Could you check a few things on this drawing? It's one solid part, dimensions in mm from its lowest x, y, z. A direction names the side the tool comes from. Round coordinates to 2 decimals unless told otherwise and drop trailing zeros. Order: outer loops, then holes, each group sorted by start corner. A loop starts at its lowest first (then second) coordinate and runs counter-clockwise, first axis right, second up. Notation, with made-up numbers: (-29, -17) -> (-6, -17) arc R10 ccw to (-6, -3) -> close; hole circle Ø5 at (59, 32). An arc over 180 degrees is marked (long way). Use a Markdown table: item, result. Add a question column.
(1) If I drill on probe 1 along Y at (x, z) = (6, 1); probe 2 along Y at (x, z) = (20, 7.75) (1 decimal); probe 3 along Y at (x, z) = (21, 3.75), over which ranges is the centre line in solid material (lowest first)?
(2) I want a section at C-C, the plane x = 14.5. Please give me the cut outline in (y, z) (1 decimal), then the cut area to 3 significant figures.
(3) I'm going to push flat-ended pins straight in: P1, Ø3, axis at x = 15, y = 24, coming from the +Z side; P2, Ø1.4, axis at x = 8.5, z = 1.5, coming from the -Y side; P3, Ø4, axis at y = 16.5, z = 3, coming from the -X side; P4, Ø4, axis at x = 11.5, y = 23, coming from the +Z side (1 decimal). Where does each tip first touch, or does it pass through?
(4) Thinking about a two-plate mould opening in Y: for the marked faces 5, 6, 7 and 8, which applies, pulls with the +Y half, pulls with the -Y half, needs draft (parallel to the pull), parting line crosses it, or undercut?
(5) On a 3-axis mill with a long thin cutter (end or side, diameter ignored), from which of +Z, -Z, +X, -X, +Y, -Y can I reach the whole of each face in a straight line? I mean the marked faces 1, 2, 3 and 4. Say none if no direction works.
(6) I want a section at A-A, the plane x = 29.5. Please give me the cut outline in (y, z).
(7) I want a section at B-B, the plane z = 11.5. Please give me the cut outline in (x, y) (1 decimal), then the cut area to 3 significant figures.
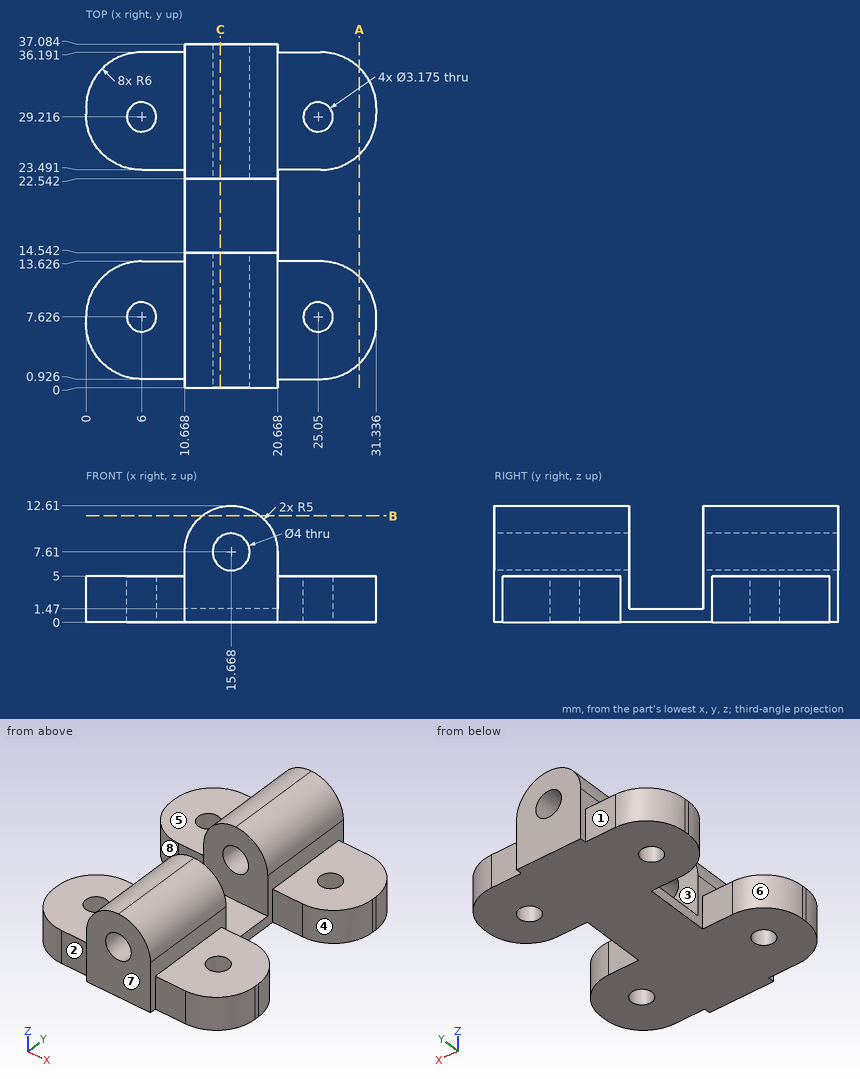
Taken from the geometry:
| question | item | result |
|---|---|---|
| 1 | probe 1 | y = 0.93 to 6.04, 9.21 to 13.63, 23.49 to 27.63, 30.8 to 36.19 |
| 1 | probe 2 | y = 0 to 14.5, 22.5 to 37.1 |
| 1 | probe 3 | y = 0.93 to 13.63, 23.49 to 36.19 |
| 2 | outline | (0, 0) -> (37.1, 0) -> (37.1, 6) -> (22.5, 6) -> (22.5, 1.5) -> (14.5, 1.5) -> (14.5, 6) -> (0, 6) -> close; (0, 9.2) -> (14.5, 9.2) -> (14.5, 12.5) -> (0, 12.5) -> close; (22.5, 9.2) -> (37.1, 9.2) -> (37.1, 12.5) -> (22.5, 12.5) -> close |
| 2 | area | 280 mm2 |
| 3 | P1 | stops at z = 12.61 |
| 3 | P2 | stops at y = 0.93 |
| 3 | P3 | stops at x = 10.67 |
| 3 | P4 | stops at z = 12.1 |
| 4 | face 5 | needs draft |
| 4 | face 6 | undercut |
| 4 | face 7 | pulls with the -Y half |
| 4 | face 8 | undercut |
| 5 | face 1 | +Z, -Z, -X, +Y |
| 5 | face 2 | +Z, -Z, -X, -Y |
| 5 | face 3 | +Z, +X, -X |
| 5 | face 4 | +Z, -Z, +X |
| 6 | outline | (2.61, 0) -> (11.95, 0) -> (11.95, 5) -> (2.61, 5) -> close; (25.17, 0) -> (34.51, 0) -> (34.51, 5) -> (25.17, 5) -> close |
| 7 | outline | (12.5, 0) -> (18.8, 0) -> (18.8, 14.5) -> (12.5, 14.5) -> close; (12.5, 22.5) -> (18.8, 22.5) -> (18.8, 37.1) -> (12.5, 37.1) -> close |
| 7 | area | 183 mm2 |
